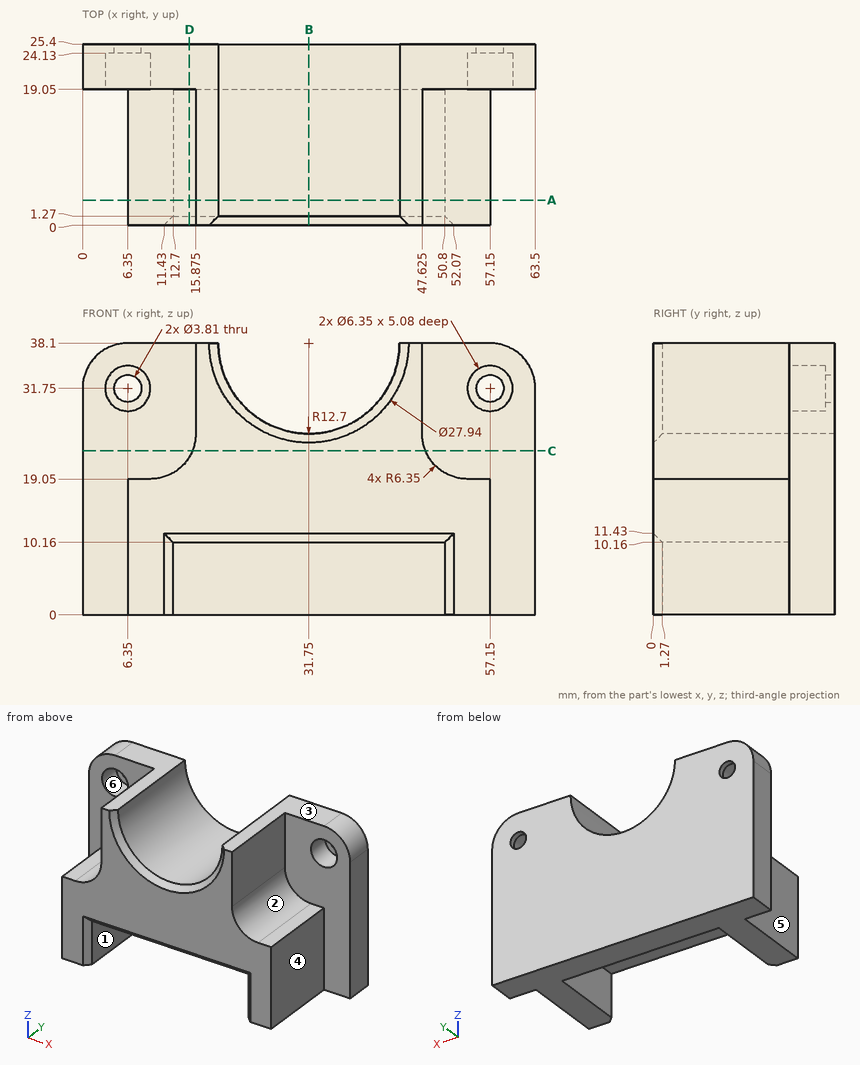
The drawing under review shows one solid part. Ordinate dimensions are in mm from its lowest x, y, z. A direction names the side the tool comes from. Coordinates: 2 decimals unless noted, no trailing zeros. Order: outer loops, then holes, each group sorted by start corner. A loop starts at its lowest first (then second) coordinate and runs counter-clockwise, first axis right, second up. Notation, with made-up numbers: (74, 85.25) -> (115, 85.25) arc R15 ccw to (115, 97.25) -> close; hole circle Ø6 at (53.25, -9.5). An arc over 180 degrees is marked (long way). Answer as CSV lines item,"result".
Q1. We need section A-A (y = 3.5). State the section outline as (x, z) points (3 decimals), plus the area to 3 significant figures.
Model answer:
outline,"(6.35, 0) -> (12.7, 0) -> (12.7, 10.16) -> (50.8, 10.16) -> (50.8, 0) -> (57.15, 0) -> (57.15, 19.05) -> (53.975, 19.05) arc R6.35 cw to (47.625, 25.4) -> (47.625, 38.1) -> (44.45, 38.1) arc R12.7 cw to (19.05, 38.1) -> (15.875, 38.1) -> (15.875, 25.4) arc R6.35 cw to (9.525, 19.05) -> (6.35, 19.05) -> close"
area,"949 mm2"
Q2. Clearance check with flat-ended pins moving along their axes: pin 1 Ø5.5 at (x, z) = (57.15, 31.75) entering from -Y; pin 2 Ø11 at (y, z) = (11.5, 5) entering from +X; pin 3 Ø1.6 at (x, y) = (55, 5.5) entering from +Z; pin 4 Ø8 at (x, y) = (23, 21) entering from +Z. State where each tip first meets the part, or that it passes through.
Model answer:
pin 1,"stops at y = 24.13"
pin 2,"stops at x = 57.15"
pin 3,"stops at z = 19.05"
pin 4,"stops at z = 38.1"
Q3. Draft analysis for pull direction X (two halves, no side actions). For the marked faces 1, 2 and 3, state which applies: released by +X, released by -X, zero draft, split by the parting line, or undercut.
Model answer:
face 1,"undercut"
face 2,"released by +X"
face 3,"zero draft"
Q4. For the marked faces 4, 5 and 6, list the 3-axis set-ups (+Z, -Z, +X, -X, +Y, -Y) from which the entire face can be reached by the end or side of a thin tool; tool diameter is ignored.
Model answer:
face 4,"+Z, -Z, +X, -Y"
face 5,"+Z, -Z, -X, -Y"
face 6,"-Y"
Q5. Wall thickness on line 1 along X through (y, z) = (7.5, 17); line 2 along Y through (x, z) = (35, 6); line 3 along Z through (x, y) = (5, 19.75): over which ranges is each line inside the solid? List them lowest first. Write a range as [from, to].
Model answer:
line 1,"x = [6.35, 57.15]"
line 2,"y = [19.05, 25.4]"
line 3,"z = [0, 28.88], [34.62, 37.95]"
Q6. We need section B-B (x = 31.75). State the section outline as (y, z) points, plus the area to 3 significant figures.
Model answer:
outline,"(0, 11.43) -> (1.27, 10.16) -> (19.05, 10.16) -> (19.05, 0) -> (25.4, 0) -> (25.4, 25.4) -> (1.27, 25.4) -> (0, 24.13) -> close"
area,"450 mm2"
Q7. We need section D-D (x = 15). State the section outline as (y, z) points, plus the area to 3 significant figures.
Model answer:
outline,"(0, 11.43) -> (1.27, 10.16) -> (19.05, 10.16) -> (19.05, 0) -> (25.4, 0) -> (25.4, 38.1) -> (19.05, 38.1) -> (19.05, 22.18) -> (0, 22.18) -> close"
area,"470 mm2"
Q8. We need section C-C (z = 23). State the section outline as (x, y) points, plus the area to 3 significant figures.
Model answer:
outline,"(0, 19.05) -> (15.4, 19.05) -> (15.4, 0) -> (48.1, 0) -> (48.1, 19.05) -> (63.5, 19.05) -> (63.5, 25.4) -> (0, 25.4) -> close"
area,"1,030 mm2"
